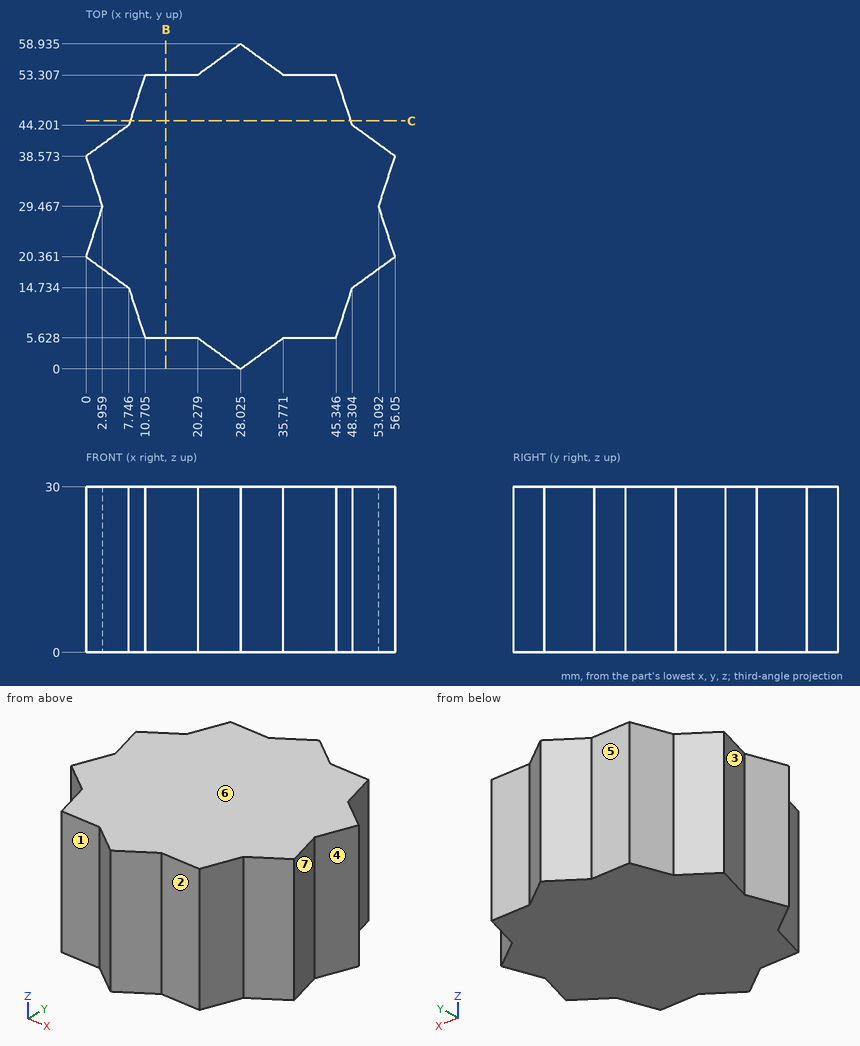
The figure shows three views and two pictorial views of one solid part (mm, origin at its lowest corner). Answer the questions. A direction names the side the tool comes from. Coordinates: 2 decimals unless noted, no trailing zeros. Write each loop counter-clockwise with the first axis right and the second up, starting at its lowest first coordinate (ties: lowest second). Pieces come first, ordered by that corner, then holes. Notation, with made-up numbers: (-2, 81.5) -> (49, 81.5) arc R31 cw to (49, 112.5) -> close; hole circle Ø8 at (43, 27.25). An arc over 180 degrees is marked (long way). Return JSON: item names as keys, results as strings.
1. Find the intervals of material crossed by line 1 along Y through (x, z) = (12, 10.25); line 2 along X through (y, z) = (28, 2); line 3 along X through (y, z) = (34, 15.25) (1 decimal), in increasing order. Write a range as from..to.
Found:
{"line 1": "5.63..53.31", "line 2": "2.48..53.57", "line 3": "1.5..54.6"}
2. A cutting plane is placed at C-C (y = 45). Determine the outline of the cut face in (x, z) (1 decimal).
Found:
{"outline": "(8, 0) -> (48, 0) -> (48, 30) -> (8, 30) -> close"}
3. Each of these flat-tipped pins is pushed along its axis until it touches: P1, Ø4, axis at y = 37.5, z = 8, coming from the +X side; P2, Ø3, axis at x = 15.5, z = 12.5, coming from the +Y side; P3, Ø6, axis at y = 25.5, z = 10.5, coming from the -X side (1 decimal); P4, Ø10, axis at x = 9.5, y = 8, coming from the +Z side. Where does it stop, or does it pass through?
Found:
{"P1": "x = 56.05", "P2": "y = 53.31", "P3": "x = 0.7", "P4": "z = 30"}
4. A cutting plane is placed at B-B (x = 14.5). Determine the outline of the cut face in (y, z).
Found:
{"outline": "(5.63, 0) -> (53.31, 0) -> (53.31, 30) -> (5.63, 30) -> close"}
5. Determine the mould class of the marked faces 5, 6 and 7 for opening direction Y: pulls with the +Y half, pulls with the -Y half, needs draft (parallel to the pull), parting line crosses it, or undercut.
Found:
{"face 5": "pulls with the +Y half", "face 6": "needs draft", "face 7": "undercut"}
6. A tool of negligible diameter and unlimited length cuts with its end or side. For the marked faces 1, 2, 3 and 4, from which of +Z, -Z, +X, -X, +Y, -Y can it reach the whole face along a straight path? Write none if from no direction.
Found:
{"face 1": "+Z, -Z, -X, -Y", "face 2": "+Z, -Z, +X, -Y", "face 3": "+Z, -Z, -X", "face 4": "+Z, -Z, +X"}
